```python
from build123d import *

# Parameters (mm, degrees)
SKETCH_1_W      = 190
SKETCH_1_H      = 105
SKETCH_1_R      = 2.5
SKETCH_1_W_2    = 20
SKETCH_1_H_2    = 41
EXTRUDE_1_DEPTH = 4
FILLET_1_R      = 5


with BuildPart() as part:
    # 草图1 → 凸台-拉伸1 (new body)
    with BuildSketch(Plane(origin=(0, 0, 0), x_dir=(1, 0, 0), z_dir=(0, 1, 0))):
        Rectangle(SKETCH_1_W, SKETCH_1_H)
        with Locations(Location((-89, 46.5, 0), (0, 0, 270))):
            Circle(SKETCH_1_R, mode=Mode.SUBTRACT)
        with Locations(Location((89, 46.5, 0), (0, 0, 270))):
            Circle(SKETCH_1_R, mode=Mode.SUBTRACT)
        with Locations(Location((-89, -46.5, 0), (0, 0, 270))):
            Circle(SKETCH_1_R, mode=Mode.SUBTRACT)
        with Locations(Location((-63, 31.5, 0), (0, 0, 270))):
            Circle(SKETCH_1_R, mode=Mode.SUBTRACT)
        with Locations(Location((33, 31.5, 0), (0, 0, 270))):
            Circle(SKETCH_1_R, mode=Mode.SUBTRACT)
        with Locations(Location((-63, -31.5, 0), (0, 0, 270))):
            Circle(SKETCH_1_R, mode=Mode.SUBTRACT)
        with Locations(Location((33, -31.5, 0), (0, 0, 270))):
            Circle(SKETCH_1_R, mode=Mode.SUBTRACT)
        with Locations(Location((63, 24.25, 0), (0, 0, 270))):
            Circle(SKETCH_1_R, mode=Mode.SUBTRACT)
        with Locations(Location((73, 24.25, 0), (0, 0, 270))):
            Circle(SKETCH_1_R, mode=Mode.SUBTRACT)
        with Locations(Location((63, -24.25, 0), (0, 0, 270))):
            Circle(SKETCH_1_R, mode=Mode.SUBTRACT)
        with Locations(Location((73, -24.25, 0), (0, 0, 270))):
            Circle(SKETCH_1_R, mode=Mode.SUBTRACT)
        with Locations(Location((46, -46.5, 0), (0, 0, 270))):
            Circle(SKETCH_1_R, mode=Mode.SUBTRACT)
        with Locations(Location((46, 46.5, 0), (0, 0, 270))):
            Circle(SKETCH_1_R, mode=Mode.SUBTRACT)
        with Locations(Location((89, -22.5, 0), (0, 0, 270))):
            Circle(SKETCH_1_R, mode=Mode.SUBTRACT)
        with Locations((68, 0)):
            Rectangle(SKETCH_1_W_2, SKETCH_1_H_2, mode=Mode.SUBTRACT)
    extrude(amount=EXTRUDE_1_DEPTH)

    # 圆角1
    fillet_1_edges = [part.edges().sort_by_distance(p)[0] for p in [
        (95, 2, 52.5),
        (-95, 2, 52.5),
        (-95, 2, -52.5),
        (95, 2, -52.5),
    ]]
    fillet(fillet_1_edges, radius=FILLET_1_R)


solid = part.part
```
Read the model definition and answer for the solid it produces. Units are mm, in the model's axes. A direction names the side the tool comes from. Give positions to 0.01 mm unless a question says otherwise; leave off trailing zeros. Write each loop counter-clockwise with the first axis right and the second up, starting at its lowest first coordinate (ties: lowest second). Pieces come first, ordered by that corner, then holes. Notation, with made-up numbers: (22, -15.75) -> (32, -15.75) arc R26 cw to (32, 16.25) -> close; hole circle Ø9 at (24.5, 30). An arc over 180 degrees is marked (long way). Answer as a JSON object with one key per item and string values.
1) For a pull along X with two mould halves and no side action, classify faces 3 (the flat face through (-1, 4, -1)), 4 (the cylindrical face through (-86.52, 1.97, 46.17)), 5 (the flat face through (95, 2, 1)), 6 (the cylindrical face through (-93.57, 2.03, 51)) as pulls with the +X half, pulls with the -X half, needs draft (parallel to the pull), parting line crosses it, or undercut.
Findings below:
{"face 3": "needs draft", "face 4": "undercut", "face 5": "pulls with the +X half", "face 6": "pulls with the -X half"}
2) Section C-C on y = 2.9 is taken. Count the separate pieces of the cut face and the enclosed holes in it, then the cut area to 3 significant figures.
Findings below:
{"separate pieces": "1", "enclosed holes": "15", "area": "18,800 mm^2"}
3) Section A-A on x = 46 is taken. Write down the section's boundary in (y, z), then the cut area to 3 significant figures.
Findings below:
{"outline": "(0, -52.5) -> (4, -52.5) -> (4, -49) -> (0, -49) -> close; (0, -44) -> (4, -44) -> (4, 44) -> (0, 44) -> close; (0, 49) -> (4, 49) -> (4, 52.5) -> (0, 52.5) -> close", "area": "380 mm^2"}
4) Section B-B on x = 73 is taken. Write down the section's boundary in (y, z).
Findings below:
{"outline": "(0, -52.5) -> (4, -52.5) -> (4, -26.75) -> (0, -26.75) -> close; (0, -21.75) -> (4, -21.75) -> (4, -20.5) -> (0, -20.5) -> close; (0, 20.5) -> (4, 20.5) -> (4, 21.75) -> (0, 21.75) -> close; (0, 26.75) -> (4, 26.75) -> (4, 52.5) -> (0, 52.5) -> close"}
5) Flat-ended cylindrical pins translate along their axes: pin 1 Ø8 at (x, z) = (-7.5, -16) entering from -Y; pin 2 Ø3 at (x, z) = (-89, 46.5) entering from +Y. Find the tip coordinate at first contact, or state that the pin passes through.
Findings below:
{"pin 1": "stops at y = 0", "pin 2": "passes through"}
6) Straight lines are drawn through the part: probe 1 along X at (y, z) = (1.8, 46.5); probe 2 along X at (y, z) = (2.5, -46.5); probe 3 along X at (y, z) = (1.25, -24.25). For each, find the intervals that lie inside material, in ascending order. Write a range as from..to.
Findings below:
{"probe 1": "x = -95..-91.5, -86.5..43.5, 48.5..95", "probe 2": "x = -95..-91.5, -86.5..43.5, 48.5..86.5, 91.5..95", "probe 3": "x = -95..60.5, 65.5..70.5, 75.5..95"}
7) A tool of negligible diameter and unlimited length cuts with its end or side. For faces 1 (the cylindrical face through (93.5, 2.03, 51.07)), 2 (the flat face through (68, 2, 20.5)), from which of +Z, -Z, +X, -X, +Y, -Y can it reach the whole face along a straight path? Write none if from no direction.
Findings below:
{"face 1": "+Z, +X, +Y, -Y", "face 2": "+Y, -Y"}
